Verification items for the finished model (mm, model axes). Face numbers are marked on the shaded views. A direction names the side the tool comes from. Give positions to 0.01 mm unless a question says otherwise; leave off trailing zeros. Write each loop counter-clockwise with the first axis right and the second up, starting at its lowest first coordinate (ties: lowest second). Pieces come first, ordered by that corner, then holes. Notation, with made-up numbers: (-19.75, 84) -> (27.25, 84) arc R16 ccw to (27.25, 93) -> close; hole circle Ø5 at (-31, 33.5). An arc over 180 degrees is marked (long way). Use one line per item in the form item = value. Start each with the question number.
(1) Section check B-B, the plane x = -46. Record the cut outline in (y, z), plus the area to 3 significant figures.
(2) Section check C-C, the plane y = 2.25. Record the cut outline in (x, z).
(3) Section check A-A, the plane x = -80. Record the cut outline in (y, z).
(4) Scan lines: L1, parallel to Y at x = -80, z = -5; L2, parallel to Z at x = -61, y = 1.5; L3, parallel to X at y = 10, z = -92.75. Record each from-to range of solid material in increasing order.
(5) Set-up check for the marked faces 1 and 2: record each of +Z, -Z, +X, -X, +Y, -Y from which the full face is reachable in a straight line by a thin tool's end or side.
(6) Section check D-D, the plane y = 8. Record the cut outline in (x, z), plus the area to 3 significant figures.
(7) Depth check by flat-ended pin: pin 1 Ø5.5 at (x, y) = (-80, 10) entering from -Z; pin 2 Ø10 at (y, z) = (6.5, -54) entering from -X; pin 3 Ø1.5 at (y, z) = (6, -70) entering from -X; pin 4 Ø10 at (y, z) = (5, -66) entering from -X. Enter the tip coordinate at first touch or a pass-through.
from build123d import *

# Parameters (mm, degrees)
BOSS_EXTRUDE1_DEPTH     = 20
CUT_EXTRUDE1_DEPTH      = 126.797456254
CUT_EXTRUDE1_DEPTH_BACK = 126.797456254
SKETCH3_R               = 3.4
CUT_EXTRUDE2_DEPTH      = 5.7
CUT_EXTRUDE3_START      = 60
CUT_EXTRUDE3_DEPTH      = 5.7
FILLET1_R               = 15
FILLET2_R               = 25


with BuildPart() as part:
    # Sketch2 → Boss-Extrude1 (new body)
    with BuildSketch(Plane(origin=(0, 0, 0), x_dir=(1, 0, 0), z_dir=(0, 1, 0))):
        Polygon((-95, 20), (-95, 0), (0, 0), (0, 100), (-95, 100), (-95, 80), (-20, 80), (-20, 20), align=None)
    extrude(amount=BOSS_EXTRUDE1_DEPTH)

    # Sketch3 → Cut-Extrude1 (cut, two sides: drawn at the far end of the back side and taken through both)
    with BuildSketch(Plane.XY.offset(-80).offset(-CUT_EXTRUDE1_DEPTH_BACK)):
        with Locations((-80, 10)):
            Circle(SKETCH3_R)
    extrude(amount=CUT_EXTRUDE1_DEPTH + CUT_EXTRUDE1_DEPTH_BACK, mode=Mode.SUBTRACT)

    # Sketch4 → Cut-Extrude2 (cut)
    with BuildSketch(Plane.XY.offset(-80)):
        Polygon((-76.175, 3.374905661), (-72.35, 10), (-76.175, 16.625094339), (-83.825, 16.625094339), (-87.65, 10), (-83.825, 3.374905661), align=None)
    extrude(amount=-CUT_EXTRUDE2_DEPTH, mode=Mode.SUBTRACT)

    # Sketch4<2> → Cut-Extrude3 (cut)
    with BuildSketch(Plane.XY.offset(-80).offset(CUT_EXTRUDE3_START)):
        Polygon((-76.175, 3.374905661), (-72.35, 10), (-76.175, 16.625094339), (-83.825, 16.625094339), (-87.65, 10), (-83.825, 3.374905661), align=None)
    extrude(amount=CUT_EXTRUDE3_DEPTH, mode=Mode.SUBTRACT)

    # Fillet1
    fillet1_edges = [part.edges().sort_by_distance(p)[0] for p in [
        (-20, 10, -20),
        (-20, 10, -80),
    ]]
    fillet(fillet1_edges, radius=FILLET1_R)

    # Fillet2
    fillet2_edges = [part.edges().sort_by_distance(p)[0] for p in [
        (0, 10, -100),
        (0, 10, 0),
    ]]
    fillet(fillet2_edges, radius=FILLET2_R)


solid = part.part
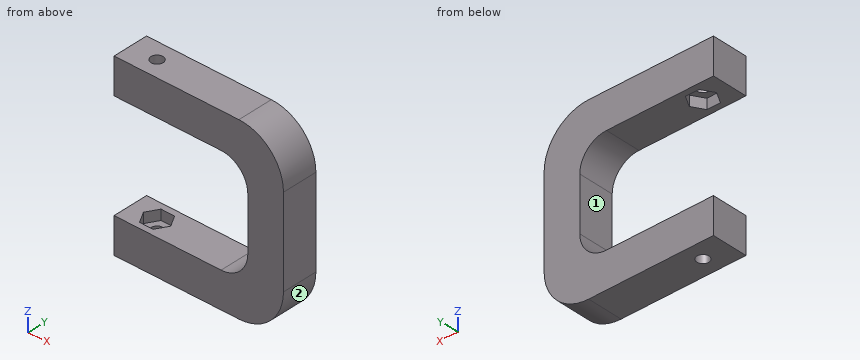
Completed:
q1.outline = (0, -100) -> (20, -100) -> (20, -80) -> (0, -80) -> close; (0, -20) -> (20, -20) -> (20, 0) -> (0, 0) -> close
q1.area = 800 mm²
q2.outline = (-95, -100) -> (-25, -100) arc R25 ccw to (0, -75) -> (0, -25) arc R25 ccw to (-25, 0) -> (-95, 0) -> (-95, -20) -> (-35, -20) arc R15 cw to (-20, -35) -> (-20, -65) arc R15 cw to (-35, -80) -> (-95, -80) -> close
q3.outline = (0, -100) -> (6.6, -100) -> (6.6, -85.7) -> (3.37, -85.7) -> (3.37, -80) -> (0, -80) -> close; (0, -20) -> (3.37, -20) -> (3.37, -14.3) -> (6.6, -14.3) -> (6.6, 0) -> (0, 0) -> close; (13.4, -100) -> (20, -100) -> (20, -80) -> (16.63, -80) -> (16.63, -85.7) -> (13.4, -85.7) -> close; (13.4, -14.3) -> (16.63, -14.3) -> (16.63, -20) -> (20, -20) -> (20, 0) -> (13.4, 0) -> close
q4.L1 = 0 to 6.6, 13.4 to 20
q4.L2 = -100 to -80, -20 to 0
q4.L3 = -95 to -83.4, -76.6 to -7.39
q5.face_1 = -X, +Y, -Y
q5.face_2 = -Z, +X, +Y, -Y
q6.outline = (-95, -100) -> (-82.75, -100) -> (-82.75, -85.7) -> (-86.5, -85.7) -> (-86.5, -80) -> (-95, -80) -> close; (-95, -20) -> (-86.5, -20) -> (-86.5, -14.3) -> (-82.75, -14.3) -> (-82.75, 0) -> (-95, 0) -> close; (-77.25, -100) -> (-25, -100) arc R25 ccw to (0, -75) -> (0, -25) arc R25 ccw to (-25, 0) -> (-77.25, 0) -> (-77.25, -14.3) -> (-73.5, -14.3) -> (-73.5, -20) -> (-35, -20) arc R15 cw to (-20, -35) -> (-20, -65) arc R15 cw to (-35, -80) -> (-73.5, -80) -> (-73.5, -85.7) -> (-77.25, -85.7) -> close
q6.area = 4,520 mm²
q7.pin_1 = through
q7.pin_2 = -20
q7.pin_3 = -21.15
q7.pin_4 = -21.25
